from build123d import *

# Parameters (mm, degrees)
BOSS_EXTRUDE1_DEPTH = 3
SKETCH2_R           = 9
SKETCH2_R_2         = 1.5
CUT_EXTRUDE1_DEPTH  = 3
SKETCH3_R           = 1.5
CUT_EXTRUDE2_DEPTH  = 12
SKETCH4_R           = 2.25
CUT_EXTRUDE3_DEPTH  = 27
SKETCH5_R           = 0.619378792
CUT_EXTRUDE4_DEPTH  = 1


with BuildPart() as part:
    # Sketch1 → Boss-Extrude1 (new body)
    with BuildSketch(Plane(origin=(0, 0, 0), x_dir=(1, 0, 0), z_dir=(0, 1, 0))):
        Polygon((9, 0), (-9, 0), (-18.5, 10.75), (-24.5, 10.75), (-24.5, 34.75), (-18.5, 34.75), (-9, 45.5), (9, 45.5), (18.5, 34.75), (32.25, 34.75), (32.25, 10.75), (18.5, 10.75), align=None)
    extrude(amount=BOSS_EXTRUDE1_DEPTH)

    # Sketch2 → Cut-Extrude1 (cut)
    with BuildSketch(Plane(origin=(0, 3, 0), x_dir=(1, 0, 0), z_dir=(0, 1, 0))):
        with Locations(Location((14, 22.75, 0), (0, 0, 270))):
            Circle(SKETCH2_R)
        with Locations(Location((-14, 22.75, 0), (0, 0, 270))):
            Circle(SKETCH2_R_2)
    extrude(amount=-CUT_EXTRUDE1_DEPTH, mode=Mode.SUBTRACT)

    # Sketch3 → Cut-Extrude2 (cut)
    with BuildSketch(Plane(origin=(0, 0, 0), x_dir=(1, 0, 0), z_dir=(0, 1, 0))):
        with Locations(Location((-5.25, 42.5, 0), (0, 0, 90))):
            Circle(SKETCH3_R)
        with Locations(Location((5.25, 42.5, 0), (0, 0, 90))):
            Circle(SKETCH3_R)
        with Locations(Location((5.25, 3, 0), (0, 0, 90))):
            Circle(SKETCH3_R)
        with Locations(Location((-5.25, 3, 0), (0, 0, 90))):
            Circle(SKETCH3_R)
    extrude(amount=CUT_EXTRUDE2_DEPTH, mode=Mode.SUBTRACT)

    # Sketch4 → Cut-Extrude3 (cut)
    with BuildSketch(Plane(origin=(0, 0, 0), x_dir=(1, 0, 0), z_dir=(0, 1, 0))):
        with Locations(Location((-20.75, 27.75, 0), (0, 0, 90))):
            Circle(SKETCH4_R)
        with Locations(Location((-20.75, 17.75, 0), (0, 0, 90))):
            Circle(SKETCH4_R)
        with Locations(Location((28.749486719, 17.75, 0), (0, 0, 90))):
            Circle(SKETCH4_R)
        with Locations(Location((28.749486719, 27.75, 0), (0, 0, 90))):
            Circle(SKETCH4_R)
    extrude(amount=CUT_EXTRUDE3_DEPTH, mode=Mode.SUBTRACT)

    # Sketch5 → Cut-Extrude4 (cut)
    with BuildSketch(Plane(origin=(0, 0, -45.5), x_dir=(-1, 0, 0), z_dir=(0, 0, -1))):
        with Locations((0, 1.5)):
            Circle(SKETCH5_R)
    extrude(amount=-CUT_EXTRUDE4_DEPTH, mode=Mode.SUBTRACT)


solid = part.part
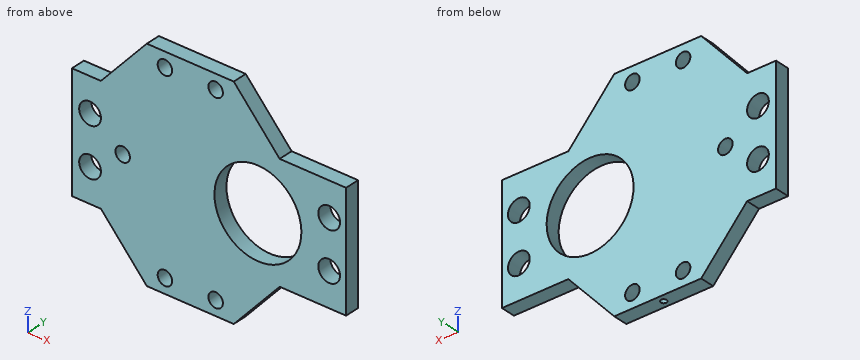
Work out the finished part from the listing and answer in its coordinate system (mm). Coordinates: 2 decimals unless noted, no trailing zeros. Write each loop counter-clockwise with the first axis right and the second up, starting at its lowest first coordinate (ties: lowest second). Pieces come first, ordered by that corner, then holes. Notation, with made-up numbers: M -35.75,46.25 L -20.75,46.25 A31 cw -20.75,82.25 Z; hole C 89.5,29.25 d2. An arc over 180 degrees is marked long. Use one line per item in the form item = value. Start each with the question number.
1. The part is cut by section D-D (x = 20.5). Give the vertices of the cut face in (y, z).
2. Straight lines are drawn through the part: probe 1 along Z at (x, y) = (4.5, 1.7); probe 2 along X at (y, z) = (1.5, -17); probe 3 along Z at (x, y) = (-5, 2.95). For each, find the intervals that lie inside material, in ascending order. Write a range as from..to.
3. The part is cut by section C-C (z = -16.5). Give the vertices of the cut face in (x, y), plus the area to 3 significant figures.
4. Each of these flat-tipped pins is pushed along its axis until it touches: P1, Ø4, axis at x = -14, z = -22.75, coming from the -Y side; P2, Ø1.5, axis at x = 19, y = 1, coming from the +Z side; P3, Ø0.9, axis at x = -21.5, y = 1, coming from the +Z side. Where does it stop, or does it pass through?
5. The part is cut by section A-A (x = -20.75). Give the vertices of the cut face in (y, z), plus the area to 3 significant figures.
6. The part is cut by section B-B (z = -22.75). Give the vertices of the cut face in (x, y).
Evaluation:
q1.outline = M 0,-34.75 L 3,-34.75 L 3,-28.97 L 0,-28.97 Z; M 0,-16.53 L 3,-16.53 L 3,-10.75 L 0,-10.75 Z
q2.probe_1 = -45.5..-43.8, -41.2..-4.3, -1.7..0
q2.probe_2 = -24.5..-22.87, -18.63..7.08, 20.92..26.63, 30.87..32.25
q2.probe_3 = -45.5..-43.98, -41.02..-4.48, -1.52..0
q3.outline = M -24.5,0 L -22.62,0 L -22.62,3 L -24.5,3 Z; M -18.88,0 L 7.52,0 L 7.52,3 L -18.88,3 Z; M 20.48,0 L 26.88,0 L 26.88,3 L 20.48,3 Z; M 30.62,0 L 32.25,0 L 32.25,3 L 30.62,3 Z
q3.area = 109 mm^2
q4.P1 = 0
q4.P2 = -10.47
q4.P3 = -10.75
q5.outline = M 0,-34.75 L 3,-34.75 L 3,-30 L 0,-30 Z; M 0,-25.5 L 3,-25.5 L 3,-20 L 0,-20 Z; M 0,-15.5 L 3,-15.5 L 3,-10.75 L 0,-10.75 Z
q5.area = 45.0 mm^2
q6.outline = M -24.5,0 L -15.5,0 L -15.5,3 L -24.5,3 Z; M -12.5,0 L 5,0 L 5,3 L -12.5,3 Z; M 23,0 L 32.25,0 L 32.25,3 L 23,3 Z
